Check sheet for the modelled part. Datum: model origin and axes. Units: mm. Round coordinates to 2 decimals unless told otherwise and drop trailing zeros. Order: outer loops, then holes, each group sorted by start corner. A loop starts at its lowest first (then second) coordinate and runs counter-clockwise, first axis right, second up.
```python
from build123d import *

# Parameters (mm, degrees)
SKETCH1_W           = 64
SKETCH1_H           = 75
BOSS_EXTRUDE1_DEPTH = 9.4
SKETCH3_R           = 0.5
BOSS_EXTRUDE2_DEPTH = 6


with BuildPart() as part:
    # Sketch1 → Boss-Extrude1 (new body)
    with BuildSketch(Plane(origin=(0, 0, 0), x_dir=(1, 0, 0), z_dir=(0, 1, 0))):
        with Locations((32, 37.5)):
            Rectangle(SKETCH1_W, SKETCH1_H)
    extrude(amount=BOSS_EXTRUDE1_DEPTH)

    # Sketch3 → Boss-Extrude2 (add)
    with BuildSketch(Plane(origin=(13.525948084, 0, 0), x_dir=(1, 0, 0), z_dir=(0, 0, 1))):
        with Locations((23.990000312, 4.397240371)):
            Circle(SKETCH3_R)
        with Locations((28.759444519, 4.234135385)):
            Circle(SKETCH3_R)
    extrude(amount=BOSS_EXTRUDE2_DEPTH)


solid = part.part
```
Item 1: Go/stop test with a flat-tipped pin: P1, Ø5, axis at x = 47, y = 6, coming from the +Z side. Record where the tip stops, or that it passes through.
Answer:
P1: stops at z = 0
Item 2: Scan line: line 1 along Z through (x, y) = (4.5, 7.5). Record every from-to range of solid material in increasing order.
Answer:
line 1: z = -75 to 0
Item 3: Sectioned sample at A-A (y = 8.5). Record the cut outline in (x, z).
Answer:
outline: (0, -75) - (64, -75) - (64, 0) - (0, 0) - close
Item 4: Sectioned sample at C-C (z = 1). Record the cut outline in (x, y).
Answer:
outline: circle Ø1 at (37.52, 4.4); circle Ø1 at (42.29, 4.23)
Item 5: Sectioned sample at B-B (x = 13). Record the cut outline in (y, z).
Answer:
outline: (0, -75) - (9.4, -75) - (9.4, 0) - (0, 0) - close
